```python
from build123d import *

# Parameters (mm, degrees)
SKETCH2_R          = 20
CUT_EXTRUDE1_DEPTH = 40


with BuildPart() as part:
    # Sketch1 → Revolve2 (revolve)
    with BuildSketch(Plane.XY, mode=Mode.PRIVATE) as revolve2_sk:
        Polygon((0, 0), (0, 25), (40, 25), (40, 35), (60, 35), (60, 25), (80, 25), (80, 20), (100, 20), (100, 15), (120, 15), (120, 10), (140, 10), (140, 5), (160, 5), (160, 0), align=None)
    revolve(revolve2_sk.sketch.rotate(Axis((0, 0, 0), (1, 0, 0)), 90), axis=Axis((0, 0, 0), (1, 0, 0)))  # turned: the seam where the file's is

    # Sketch2 → Cut-Extrude1 (cut)
    with BuildSketch(Plane.ZY):
        Circle(SKETCH2_R)
    extrude(amount=-CUT_EXTRUDE1_DEPTH, mode=Mode.SUBTRACT)


solid = part.part
```
Check sheet for the modelled part. Datum: model origin and axes. Units: mm. A direction names the side the tool comes from. Coordinates: 2 decimals unless noted, no trailing zeros. Write each loop counter-clockwise with the first axis right and the second up, starting at its lowest first coordinate (ties: lowest second). Pieces come first, ordered by that corner, then holes. Notation, with made-up numbers: (-36.5, -14.75) - (-0.5, -14.75) arc R22 cw to (-0.5, -3.75) - close; hole circle Ø6 at (82.5, 49). An arc over 180 degrees is marked (long way). One line per question, with ' | ' between items.
Item 1: Mould release check, pull along Y, two halves, no side actions. Record for faces 1 (the face through (160, 0, 0)), 2 (the face through (110.14, -12.65, 8.06)), 3 (the face through (40, 0, 0)): pulls with the +Y half, pulls with the -Y half, needs draft (parallel to the pull), parting line crosses it, or undercut.
Determined:
face 1: needs draft | face 2: parting line crosses it | face 3: undercut
Item 2: Gauge pin test, flat ends, axial feed: P1, Ø1.5, axis at x = 129, z = 3.5, coming from the +Y side; P2, Ø12, axis at y = -9.5, z = 2, coming from the -X side; P3, Ø8, axis at x = 110.5, y = 9, coming from the +Z side. Record the tip position at first contact, or that the pin passes through.
Determined:
P1: stops at y = 9.61 | P2: stops at x = 40 | P3: stops at z = 14.14
Item 3: Sectioned sample at D-D on x = 71. Record the boundary of the cut face in (y, z).
Determined:
outline: circle Ø50 at (0, 0)
Item 4: Sectioned sample at C-C on x = 94. Record the boundary of the cut face in (y, z).
Determined:
outline: circle Ø40 at (0, 0)
Item 5: Access from +Z, -Z, +X, -X, +Y, -Y to the whole of each face (thin tool, end or side, straight path). Record for faces 4 (the face through (80, -17, -11)), 5 (the face through (19.72, -19.524, -4.336)), 6 (the face through (0, -17, 11)).
Determined:
face 4: +X | face 5: -X | face 6: +Z, -Z, -X, +Y, -Y
Item 6: Thickness scan on line 1 (Y direction, x = 22.5, z = 0); line 2 (X direction, y = -2.5, z = 18); line 3 (X direction, y = -11, z = 17.5). Record the ranges inside material, lowest first. Write a range as [from, to].
Determined:
line 1: y = [-25, -20], [20, 25] | line 2: x = [40, 100] | line 3: x = [0, 80]
